Autodesk Inventor part; units mm, degrees
ref_plane "YZ Plane" through (0, 0, 0) normal (1, 0, 0) x (0, 1, 0)
ref_plane "XZ Plane" through (0, 0, 0) normal (0, 1, 0) x (-1, 0, 0)
ref_plane "XY Plane" through (0, 0, 0) normal (0, 0, 1) x (1, 0, 0)
sketch "Sketch1" plane through (0, 0, 0) normal (0, 1, 0) x (-1, 0, 0)
  line L0 (3.175, 0) -> (9.525, 0)
  line L1 (12.7, 3.175) -> (12.7, 200.025)
  line L2 (9.525, 203.2) -> (3.175, 203.2)
  line L3 (0, 200.025) -> (0, 3.175)
  circle A0 centre (6.35, 196.85) radius 2.5797
  circle A1 centre (6.35, 6.35) radius 2.5797
  arc A2 (12.7, 200.025) -> (9.525, 203.2) centre (9.525, 200.025) ccw
  arc A3 (3.175, 203.2) -> (0, 200.025) centre (3.175, 200.025) ccw
  arc A4 (0, 3.175) -> (3.175, 0) centre (3.175, 3.175) ccw
  arc A5 (9.525, 0) -> (12.7, 3.175) centre (9.525, 3.175) ccw
  point P0 (0, 0)
  point P1 (12.7, 203.2)
  point P2 (0, 203.2)
  dimension "d0" = 12.7
  dimension "d1" = 5.1594
  dimension "d2" = 6.35
  dimension "d3" = 6.35
  dimension "d4" = 6.35
  dimension "d5" = 6.35
  dimension "d6" = 203.2
  dimension "d7" = 3.175
extrude "Extrusion1" add sketch "Sketch1" along normal blind 9.525
equation "\"d2\" = 0.5 * d0"
equation "\"d3\" = d2"
equation "\"d4\" = d2"
equation "\"d5\" = d3"
properties part number "Inner swing"
The listing builds one solid part. Answer for the finished solid, in the listing's coordinates (mm). Round coordinates to 2 decimals unless told otherwise and drop trailing zeros. Order: outer loops, then holes, each group sorted by start corner. A loop starts at its lowest first (then second) coordinate and runs counter-clockwise, first axis right, second up. Notation, with made-up numbers: (53.5, 78.5) - (59.5, 78.5) arc R25 cw to (59.5, 115.5) - close; hole circle Ø9 at (85, 81.25). An arc over 180 degrees is marked (long way). Put each result on its own line as item: value. Start each with the question number.
(1) Determine the mould class of faces 1 (the flat face through (-12.7, 5, 100)), 2 (the flat face through (-6, 0, 103)), 3 (the cylindrical face through (-6.014, 4.696, 194.292)), 4 (the cylindrical face through (-7.737, 4.696, 4.175)) for opening direction X: released by +X, released by -X, zero draft, split by the parting line, or undercut.
(2) Find section C-C (y = 4). Give the vertices of the cut face in (x, z) (3 decimals), plus the area to 3 significant figures.
(3) Find section A-A (z = 196.85). Give the vertices of the cut face in (x, y) (3 decimals), plus the area to 3 significant figures.
(4) Straight lines are drawn through the part: probe 1 along Z at (x, y) = (-6.35, 2.25); probe 2 along Z at (x, y) = (-4.75, 8); probe 3 along X at (y, z) = (2.25, 196.85). For each, find the intervals that lie inside material, in ascending order. Write a range as from..to.
(5) Find section B-B (x = -6.35). Give the vertices of the cut face in (y, z) (3 decimals).
Reply:
1. face 1: released by -X
1. face 2: zero draft
1. face 3: undercut
1. face 4: undercut
2. outline: (-12.7, 3.175) arc R3.175 ccw to (-9.525, 0) - (-3.175, 0) arc R3.175 ccw to (0, 3.175) - (0, 200.025) arc R3.175 ccw to (-3.175, 203.2) - (-9.525, 203.2) arc R3.175 ccw to (-12.7, 200.025) - close; hole circle Ø5.159 at (-6.35, 6.35); hole circle Ø5.159 at (-6.35, 196.85)
2. area: 2,530 mm^2
3. outline: (-12.7, 0) - (-8.93, 0) - (-8.93, 9.525) - (-12.7, 9.525) - close; (-3.77, 0) - (0, 0) - (0, 9.525) - (-3.77, 9.525) - close
3. area: 71.8 mm^2
4. probe 1: 0..3.77, 8.93..194.27, 199.43..203.2
4. probe 2: 0..4.33, 8.37..194.83, 198.87..203.2
4. probe 3: -12.7..-8.93, -3.77..0
5. outline: (0, 0) - (9.525, 0) - (9.525, 3.77) - (0, 3.77) - close; (0, 8.93) - (9.525, 8.93) - (9.525, 194.27) - (0, 194.27) - close; (0, 199.43) - (9.525, 199.43) - (9.525, 203.2) - (0, 203.2) - close
